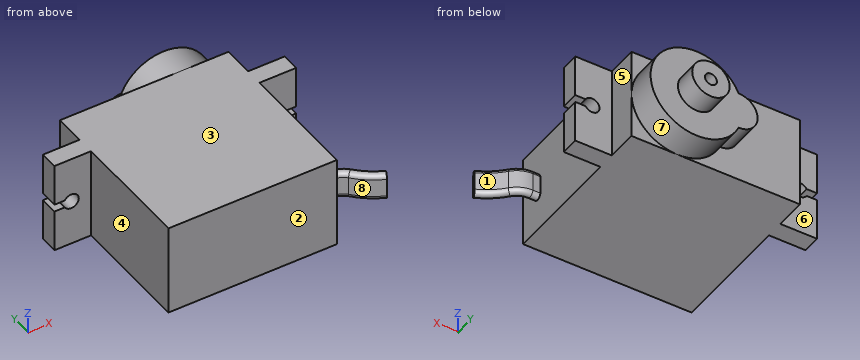
from build123d import *

# Parameters (mm, degrees)
SKETCH1_R               = 6.15
BOSS_EXTRUDE1_DEPTH     = 4
SKETCH2_W               = 22.5
SKETCH2_H               = 12.3
BOSS_EXTRUDE2_DEPTH     = 4.1
BOSS_EXTRUDE3_DEPTH     = 2.4
SKETCH4_W               = 22.5
SKETCH4_H               = 12.3
BOSS_EXTRUDE4_DEPTH     = 23
CUT_EXTRUDE1_DEPTH      = 39.381017444
CUT_EXTRUDE1_DEPTH_BACK = 39.381017444
SKETCH6_R               = 2.5
BOSS_EXTRUDE5_DEPTH     = 23
SKETCH7_R               = 2.5
SKETCH7_R_2             = 0.8
BOSS_EXTRUDE6_DEPTH     = 3
SCALE1_SCALE            = 2


with BuildPart() as part:
    # Sketch1 → Boss-Extrude1 (new body)
    with BuildSketch(Plane(origin=(0, 0, 0), x_dir=(1, 0, 0), z_dir=(0, 1, 0))):
        with Locations(Location((0, 0, 0), (0, 0, 270))):
            Circle(SKETCH1_R)
    extrude(amount=BOSS_EXTRUDE1_DEPTH)

    # Sketch2 → Boss-Extrude2 (add)
    with BuildSketch(Plane(origin=(0, 0, 0), x_dir=(1, 0, 0), z_dir=(0, 1, 0))):
        with Locations((-5.1, 0)):
            Rectangle(SKETCH2_W, SKETCH2_H)
    extrude(amount=-BOSS_EXTRUDE2_DEPTH)

    # Sketch3 → Boss-Extrude3 (add)
    with BuildSketch(Plane.XZ.offset(4.1)):
        with BuildLine():
            Line((-21.25, 6.15), (11.05, 6.15))
            Line((11.05, 6.15), (11.05, 0.5))
            Line((11.05, 0.5), (9.666025404, 0.5))
            ThreePointArc((9.666025404, 0.5), (7.8, 0), (9.666025404, -0.5))
            Line((9.666025404, -0.5), (11.05, -0.5))
            Line((11.05, -0.5), (11.05, -6.15))
            Line((11.05, -6.15), (-21.25, -6.15))
            Line((-21.25, -6.15), (-21.25, -0.5))
            Line((-21.25, -0.5), (-19.866025404, -0.5))
            ThreePointArc((-19.866025404, -0.5), (-18, 0), (-19.866025404, 0.5))
            Line((-19.866025404, 0.5), (-21.25, 0.5))
            Line((-21.25, 0.5), (-21.25, 6.15))
        make_face()
    extrude(amount=BOSS_EXTRUDE3_DEPTH)

    # Sketch4 → Boss-Extrude4 (add)
    with BuildSketch(Plane.XZ.offset(6.5)):
        with Locations((-5.1, 0)):
            Rectangle(SKETCH4_W, SKETCH4_H)
    extrude(amount=BOSS_EXTRUDE4_DEPTH)

    # Sketch5 → Cut-Extrude1 (cut, two sides: drawn at the far end of the back side and taken through both)
    with BuildSketch(Plane.XY.offset(6.15).offset(-CUT_EXTRUDE1_DEPTH_BACK)):
        Polygon((113.386591398, -22.7), (14.208205906, -22.7), (-24.661428279, -22.7), (-123.83981377, -22.7), (-123.83981377, -221.056770983), (113.386591398, -221.056770983), align=None)
    extrude(amount=CUT_EXTRUDE1_DEPTH + CUT_EXTRUDE1_DEPTH_BACK, mode=Mode.SUBTRACT)

    # Sketch6 → Boss-Extrude5 (add)
    with BuildSketch(Plane(origin=(0, 4, 0), x_dir=(1, 0, 0), z_dir=(0, 1, 0))):
        with Locations((-5.65, 0)):
            Circle(SKETCH6_R)
    extrude(amount=-BOSS_EXTRUDE5_DEPTH)

    # Sketch7 → Boss-Extrude6 (add)
    with BuildSketch(Plane(origin=(0, 4, 0), x_dir=(1, 0, 0), z_dir=(0, 1, 0))):
        with Locations(Location((0, 0, 0), (0, 0, 270))):
            Circle(SKETCH7_R)
        with Locations(Location((0, 0, 0), (0, 0, 270))):
            Circle(SKETCH7_R_2, mode=Mode.SUBTRACT)
    extrude(amount=BOSS_EXTRUDE6_DEPTH)

    # Sweep1: sweep along a path in Sketch9
    with BuildLine(Plane.XY) as sweep1_path:
        Line((6.15, -19.7), (7.149053508, -19.7))
        ThreePointArc((7.149053508, -19.7), (8.291747726, -19.944708597), (9.23401566, -20.63591299))
        ThreePointArc((9.23401566, -20.63591299), (10.752004703, -22.013665811), (12.527651525, -23.038151992))
    # Sketch8 → Sweep1 (sweep)
    with BuildSketch(Plane(origin=(6.15, 0, 0), x_dir=(0, 0, -1), z_dir=(1, 0, 0))):
        with BuildLine():
            Line((-1.2, -19.1), (1.2, -19.1))
            ThreePointArc((1.2, -19.1), (1.8, -19.7), (1.2, -20.3))
            Line((1.2, -20.3), (-1.2, -20.3))
            ThreePointArc((-1.2, -20.3), (-1.8, -19.7), (-1.2, -19.1))
        make_face()
    sweep(path=sweep1_path.line)


with BuildPart() as part_1:
    # Scale1: scaled about (-4.670030393, -10.089014718, 0)
    add(part.part.scale(SCALE1_SCALE).moved(Location((4.670030393, 10.089014718, 0))))


solid = part_1.part
Part model, mm, in its own coordinate system. Face numbers are marked on the shaded views. A direction names the side the tool comes from. Give positions to 0.01 mm unless a question says otherwise; leave off trailing zeros. Write each loop counter-clockwise with the first axis right and the second up, starting at its lowest first coordinate (ties: lowest second). Pieces come first, ordered by that corner, then holes.
1) Cut at D-D on x = 12. Write the cut outline in (y, z).
Resolved:
outline: (-35.31, -12.3) - (10.09, -12.3) - (10.09, -9.88) - (18.09, -9.88) - (18.09, 9.88) - (10.09, 9.88) - (10.09, 12.3) - (-35.31, 12.3) - close
2) Pin check, flat tips, straight feed: pin 1 (1 mm diameter, centred on y = -29, z = -1.5, fed in from -X); pin 2 (3.5 mm diameter, centred on x = 22.27, z = 0, fed in from -Y); pin 3 (12 mm diameter, centred on x = -6.5, z = -6, fed in from -Y); pin 4 (12.5 mm diameter, centred on x = 8.5, z = 5.5, fed in from +Y). Stop position of each tip, or through.
Resolved:
pin 1: stops at x = -28.03
pin 2: stops at y = -33.75
pin 3: stops at y = -35.31
pin 4: stops at y = 24.09
3) Cut at C-C on y = 9. Write the cut outline in (x, z).
Resolved:
outline: (-28.03, -12.3) - (16.97, -12.3) - (16.97, 12.3) - (-28.03, 12.3) - close
4) Probe L1, parallel to Y at x = -23, z = -4.5; L2, parallel to Y at x = 25.5, z = -5; L3, parallel to X at y = -10.5, z = 2. List the from-to ranges inside material, lowest first.
Resolved:
L1: y = -35.31 to 10.09
L2: y = -2.91 to 1.89
L3: x = -28.03 to 16.97
5) Cut at A-A on x = -16.5. Write the cut outline in (y, z).
Resolved:
outline: (-35.31, -12.3) - (10.09, -12.3) - (10.09, 12.3) - (-35.31, 12.3) - close
6) Cut at B-B on z = 8.25. Write the cut outline in (x, y), then the cut area to 3 significant figures.
Resolved:
outline: (-37.83, -2.91) - (-28.03, -2.91) - (-28.03, -35.31) - (16.97, -35.31) - (16.97, -2.91) - (26.77, -2.91) - (26.77, 1.89) - (16.97, 1.89) - (16.97, 10.09) - (13.79, 10.09) - (13.79, 18.09) - (-4.45, 18.09) - (-4.45, 10.09) - (-28.03, 10.09) - (-28.03, 1.89) - (-37.83, 1.89) - close
area: 2,280 mm2
7) Which spindle directions (+Z, -Z, +X, -X, +Y, -Y) get a long thin tool onto all of the face, cutting with end or side? Do the marked faces 4, 5, 6, 7 and 8. Say none if no direction does.
Resolved:
face 4: +Z, -Z, -X, -Y
face 5: +Z, -Z, +X, +Y
face 6: +Z, -Z, -X, +Y
face 7: +Y
face 8: +Z, -Z, -Y
8) Two-plate mould, pull along Y, no slides. Class the marked faces 1, 2 and 3: released by +Y, released by -Y, zero draft, split by the parting line, or undercut.
Resolved:
face 1: undercut
face 2: released by -Y
face 3: zero draft
